Check sheet for the drawn part. Datum: minimum x, y, z corner. Units: mm. A direction names the side the tool comes from. Give positions to 0.01 mm unless a question says otherwise; leave off trailing zeros. Write each loop counter-clockwise with the first axis right and the second up, starting at its lowest first coordinate (ties: lowest second). Pieces come first, ordered by that corner, then holes. Notation, with made-up numbers: (-27.5, 13) -> (24.5, 13) arc R31 cw to (24.5, 43) -> close; hole circle Ø10 at (52.5, -32). An arc over 180 degrees is marked (long way). Answer as CSV lines item,"result". Start each with the question number.
1) Sectioned sample at C-C on y = 32. Record the cut outline in (x, z).
2) Sectioned sample at D-D on x = 44. Record the cut outline in (y, z).
3) Sectioned sample at B-B on z = 21. Record the cut outline in (x, y), and give its area (3 significant figures).
4) Sectioned sample at A-A on x = 24. Record the cut outline in (y, z).
5) Gauge pin test, flat ends, axial feed: pin 1 Ø7 at (x, z) = (24, 21) entering from +Y; pin 2 Ø1.5 at (x, z) = (27, 5) entering from -Y; pin 3 Ø21.5 at (x, z) = (21, 24) entering from +Y; pin 4 Ø3 at (y, z) = (20.5, 8) entering from +X. Record the tip position at first contact, or that the pin passes through.
6) Material ranges on L1, parallel to Y at x = 46, z = 21; L2, parallel to Z at x = 24, y = 15.75; L3, parallel to X at y = 11, z = 21, recorded low to high.
7) Mould release check, pull along X, two halves, no side actions. Record for the marked faces 1, 2, 3 and 4: released by +X, released by -X, zero draft, split by the parting line, or undercut.
8) Tool access check on the marked faces 5, 6 and 7. Record the directions out of +Z, -Z, +X, -X, +Y, -Y that give a thin tool (end or side, any length) a straight path to the whole face; none if there is none.
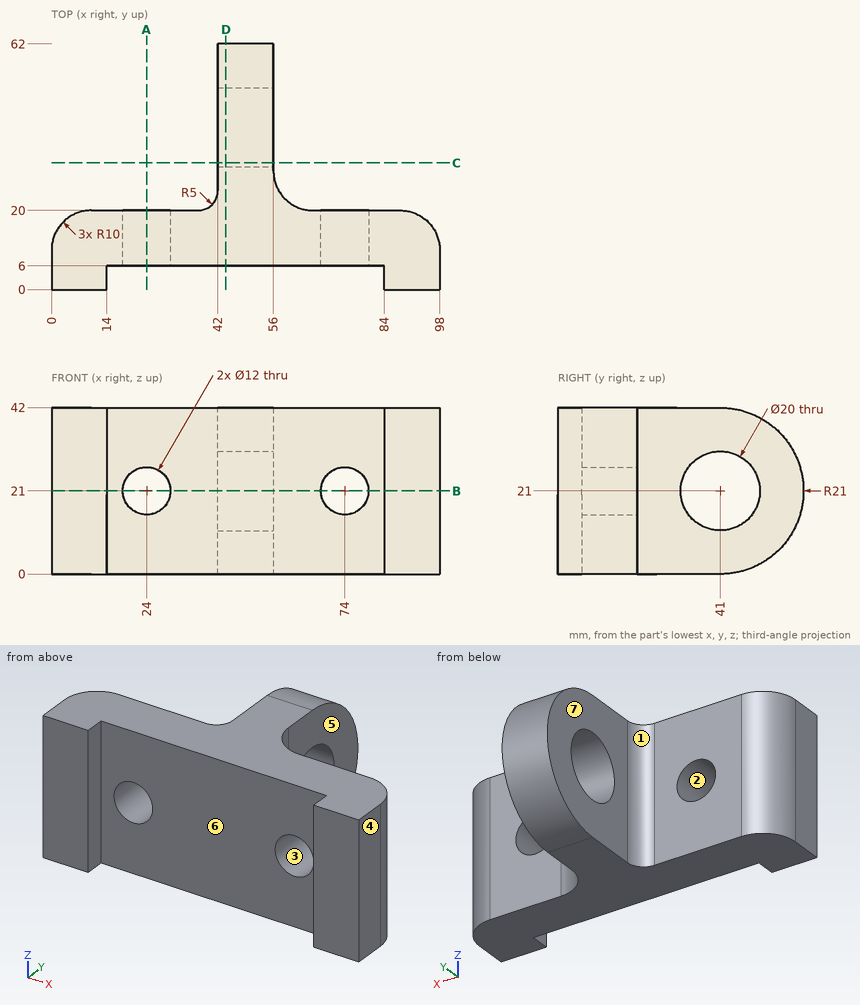
Ans:
1,outline,"(42, 0) -> (56, 0) -> (56, 16.64) -> (42, 16.64) -> close; (42, 25.36) -> (56, 25.36) -> (56, 42) -> (42, 42) -> close"
2,outline,"(6, 0) -> (41, 0) arc R21 ccw to (41, 42) -> (6, 42) -> close; hole circle Ø20 at (41, 21)"
3,outline,"(0, 0) -> (14, 0) -> (14, 6) -> (18, 6) -> (18, 20) -> (10, 20) arc R10 ccw to (0, 10) -> close; (30, 6) -> (68, 6) -> (68, 20) -> (66, 20) arc R10 cw to (56, 30) -> (56, 31) -> (42, 31) -> (42, 25) arc R5 cw to (37, 20) -> (30, 20) -> close; (42, 51) -> (56, 51) -> (56, 62) -> (42, 62) -> close; (80, 6) -> (84, 6) -> (84, 0) -> (98, 0) -> (98, 10) arc R10 ccw to (88, 20) -> (80, 20) -> close"
3,area,"1,500 mm²"
4,outline,"(6, 0) -> (20, 0) -> (20, 15) -> (6, 15) -> close; (6, 27) -> (20, 27) -> (20, 42) -> (6, 42) -> close"
5,pin 1,"passes through"
5,pin 2,"stops at y = 6"
5,pin 3,"stops at y = 20"
5,pin 4,"stops at x = 92.36"
6,L1,"y = 6 to 31, 51 to 62"
6,L2,"z = 0 to 15, 27 to 42"
6,L3,"x = 0.05 to 18, 30 to 68, 80 to 97.95"
7,face 1,"released by -X"
7,face 2,"undercut"
7,face 3,"undercut"
7,face 4,"released by +X"
8,face 5,"+Z, -Z, +X, +Y"
8,face 6,"+Z, -Z, -Y"
8,face 7,"+Z, -Z, -X, +Y"
